Geometry check sheet. Reference: drawing and pictorial views, mm from the part's lowest x, y, z. Round coordinates to 2 decimals unless told otherwise and drop trailing zeros. Order: outer loops, then holes, each group sorted by start corner. A loop starts at its lowest first (then second) coordinate and runs counter-clockwise, first axis right, second up. Notation, with made-up numbers: M -36.5,36.25 L -9.5,36.25 A14 ccw -9.5,56.25 Z; hole C 10.5,-37 d3. An arc over 180 degrees is marked long. Answer as a JSON object with one key per item and string values. Group by question number.
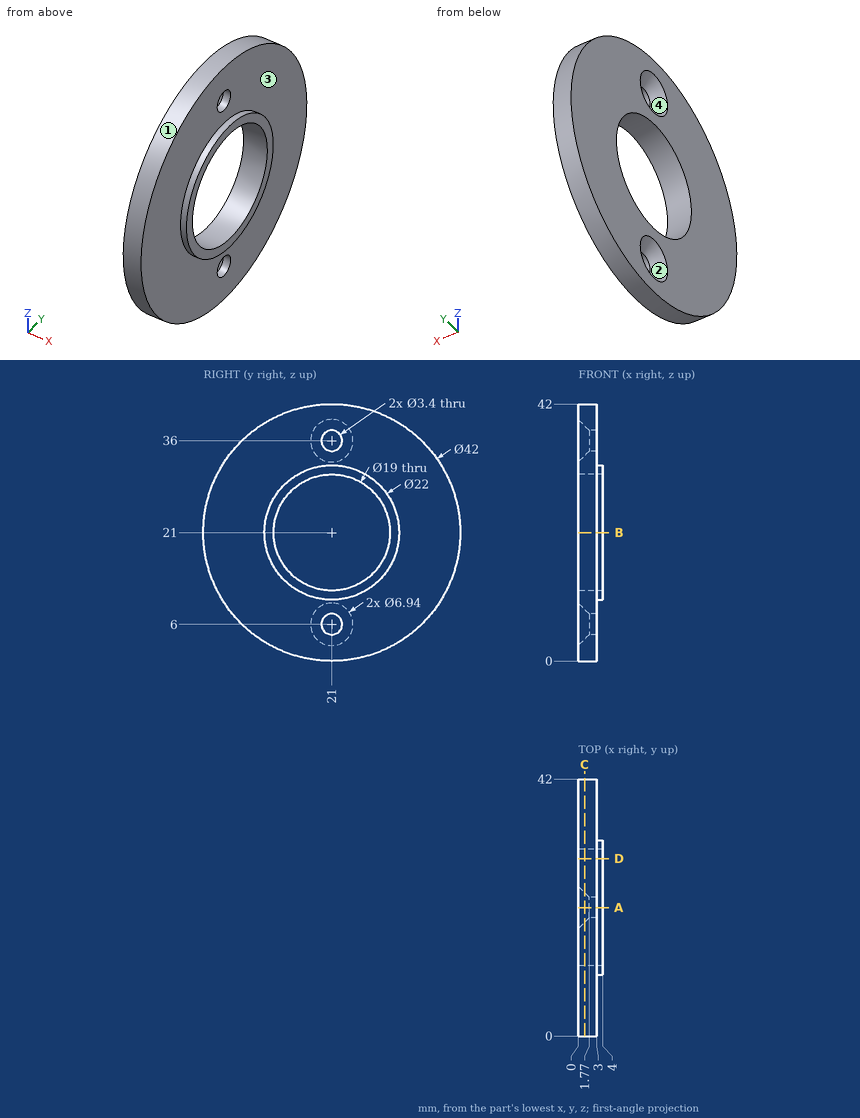
Q1. Cross-section at C-C, the plane x = 1.05. Record the cut outline in (y, z).
Q2. Gauge pin test, flat ends, axial feed: pin 1 Ø3 at (y, z) = (21, 6) entering from -X; pin 2 Ø1 at (x, y) = (0.5, 37.5) entering from -Z. Record the tip position at first contact, or that the pin passes through.
Q3. Cross-section at B-B, the plane z = 21. Record the cut outline in (x, y), then the cut area to 3 significant figures.
Q4. Release check for a two-part mould opening along Y. For the marked faces 1, 2, 3 and 4 record: released by +Y, released by -Y, zero draft, split by the parting line, or undercut.
Q5. Cross-section at A-A, the plane y = 21. Record the cut outline in (x, z).
Q6. Thickness scan on line 1 (Z direction, x = 2.65, y = 21); line 2 (Y direction, x = 2.9, z = 21); line 3 (X direction, y = 7, z = 31.5). Record the ranges inside material, lowest first. Write a range as from..to.
Q7. Cross-section at D-D, the plane y = 29. Record the cut outline in (x, z).
Conclusion:
{
 "1": {"outline": "C 21,21 d42; hole C 21,21 d19; hole C 21,6 d4.84; hole C 21,36 d4.84"},
 "2": {"pin 1": "through", "pin 2": "z = 7.4"},
 "3": {"outline": "M 0,0 L 3,0 L 3,10 L 4,10 L 4,11.5 L 0,11.5 Z; M 0,30.5 L 4,30.5 L 4,32 L 3,32 L 3,42 L 0,42 Z", "area": "72.0 mm2"},
 "4": {"face 1": "split by the parting line", "face 2": "undercut", "face 3": "zero draft", "face 4": "undercut"},
 "5": {"outline": "M 0,0 L 3,0 L 3,4.3 L 1.77,4.3 L 0,2.53 Z; M 0,9.47 L 1.77,7.7 L 3,7.7 L 3,10 L 4,10 L 4,11.5 L 0,11.5 Z; M 0,30.5 L 4,30.5 L 4,32 L 3,32 L 3,34.3 L 1.77,34.3 L 0,32.53 Z; M 0,39.47 L 1.77,37.7 L 3,37.7 L 3,42 L 0,42 Z"},
 "6": {"line 1": "0..4.3, 7.7..11.5, 30.5..34.3, 37.7..42", "line 2": "0..11.5, 30.5..42", "line 3": "0..3"},
 "7": {"outline": "M 0,1.58 L 3,1.58 L 3,13.45 L 4,13.45 L 4,15.88 L 0,15.88 Z; M 0,26.12 L 4,26.12 L 4,28.55 L 3,28.55 L 3,40.42 L 0,40.42 Z"}
}
